Here's how the part is built. I have some questions about the finished solid (model axes, mm). A direction names the side the tool comes from. Give positions to 0.01 mm unless a question says otherwise; leave off trailing zeros. Order: outer loops, then holes, each group sorted by start corner. A loop starts at its lowest first (then second) coordinate and runs counter-clockwise, first axis right, second up. Notation, with made-up numbers: (-40, 61) -> (5, 61) arc R20 cw to (5, 69) -> close; hole circle Ø11 at (0.25, -12). An arc over 180 degrees is marked (long way). Write each question's results on one line, items separated by ' | '. Start each with the question number.
Q1. Thinking about a two-plate mould opening in X: for faces 4 (the face through (-13.715, -4, -7)), 5 (the face through (5, -33.779, -7)), 6 (the face through (5, 27.921, -7)), 7 (the face through (16, -23, 0)), which applies, pulls with the +X half, pulls with the -X half, needs draft (parallel to the pull), parting line crosses it, or undercut?
Q2. I need wall thicknesses on line 1 along Y through (x, z) = (16, -3.25); line 2 along X through (y, z) = (-27, -8.25); line 3 along Y through (x, z) = (7, -3.25). Which ranges of each line are inside material? Lowest first, please. Write a range as [from, to].
Q3. For faces 1 (the face through (14.75, -26.114, 1.507)), 2 (the face through (5, -35.779, -7)), 3 (the face through (20.585, -4, -7)), which set-ups out of +Z, -Z, +X, -X, +Y, -Y let a thin tool reach every point of the face, with its end or its side?
Q4. I'm going to push flat-ended pins straight in: pin 1 (1.4 mm diameter, centred on x = -6, y = 22.5, fed in from -Z); pin 2 (1.4 mm diameter, centred on x = -7, y = -24, fed in from +Z); pin 3 (3 mm diameter, centred on x = 14, y = 13, fed in from -Z). Where does each tip first touch, or does it pass through?
Q5. Imagine slicing it at B-B, the plane z = -5.75. Please give me the cut outline in (x, y).
Q6. Imagine slicing it at D-D, the plane y = -1. Please give me the cut outline in (x, z), then the cut area to 3 significant figures.
```python
from build123d import *

# Parameters (mm, degrees)
CROQUIS1_W              = 36.3
CROQUIS1_H              = 63.7
SALIENTE_EXTRUIR1_DEPTH = 2
CROQUIS2_R              = 1.45
CORTAR_EXTRUIR1_DEPTH   = 43.35833467
CROQUIS3_W              = 36.3
CROQUIS3_H              = 63.7
CROQUIS3_W_2            = 32.3
CROQUIS3_H_2            = 59.7
SALIENTE_EXTRUIR2_DEPTH = 15
CROQUIS4_W              = 8.458215844
CROQUIS4_H              = 3.322323253
CORTAR_EXTRUIR2_DEPTH   = 15
CROQUIS5_W              = 10.947551138
CROQUIS5_H              = 4.889557179
CORTAR_EXTRUIR3_DEPTH   = 1
CROQUIS6_R              = 2.4
SALIENTE_EXTRUIR3_DEPTH = 10
REDONDEO1_R             = 1
CORTAR_EXTRUIR4_DEPTH   = 1


with BuildPart() as part:
    # Croquis1 → Saliente-Extruir1 (new body)
    with BuildSketch(Plane.XY):
        with Locations((4.435020115, -3.929119363)):
            Rectangle(CROQUIS1_W, CROQUIS1_H)
    extrude(amount=SALIENTE_EXTRUIR1_DEPTH)

    # Croquis2 → Cortar-Extruir1 (cut, through all)
    with BuildSketch(Plane(origin=(0, 0, 0), x_dir=(-1, 0, 0), z_dir=(0, 0, -1))):
        with Locations((-16.185020115, 23.120880637)):
            Circle(CROQUIS2_R)
        with Locations((7.314979885, 23.120880637)):
            Circle(CROQUIS2_R)
        with Locations((7.314979885, -23.479119363)):
            Circle(CROQUIS2_R)
        with Locations((-16.185020115, -23.479119363)):
            Circle(CROQUIS2_R)
    extrude(amount=-CORTAR_EXTRUIR1_DEPTH, mode=Mode.SUBTRACT)

    # Croquis3 → Saliente-Extruir2 (add)
    with BuildSketch(Plane(origin=(0, 0, 0), x_dir=(-1, 0, 0), z_dir=(0, 0, -1))):
        with Locations((-4.435020115, -3.929119363)):
            Rectangle(CROQUIS3_W, CROQUIS3_H)
        with Locations((-4.435020115, -3.929119363)):
            Rectangle(CROQUIS3_W_2, CROQUIS3_H_2, mode=Mode.SUBTRACT)
    extrude(amount=SALIENTE_EXTRUIR2_DEPTH)

    # Croquis4 → Cortar-Extruir2 (cut)
    with BuildSketch(Plane(origin=(0, 27.920880637, 0), x_dir=(1, 0, 0), z_dir=(0, 1, 0))):
        with Locations((4.530912193, 12.938838374)):
            Rectangle(CROQUIS4_W, CROQUIS4_H)
    extrude(amount=-CORTAR_EXTRUIR2_DEPTH, mode=Mode.SUBTRACT)

    # Croquis5 → Cortar-Extruir3 (cut)
    with BuildSketch(Plane(origin=(0, 27.920880637, 0), x_dir=(1, 0, 0), z_dir=(0, 1, 0))):
        with Locations((4.498418707, 12.555221411)):
            Rectangle(CROQUIS5_W, CROQUIS5_H)
    extrude(amount=-CORTAR_EXTRUIR3_DEPTH, mode=Mode.SUBTRACT)

    # Croquis6 → Saliente-Extruir3 (add)
    with BuildSketch(Plane(origin=(0, 0, 0), x_dir=(-1, 0, 0), z_dir=(0, 0, -1))):
        with Locations(Location((-16.185020115, 23.120880637, 0), (0, 0, 180))):
            Circle(CROQUIS6_R)
        with Locations(Location((7.314979885, 23.120880637, 0), (0, 0, 180))):
            Circle(CROQUIS6_R)
        with Locations(Location((7.314979885, -23.479119363, 0), (0, 0, 180))):
            Circle(CROQUIS6_R)
        with Locations(Location((-16.185020115, -23.479119363, 0), (0, 0, 180))):
            Circle(CROQUIS6_R)
    extrude(amount=SALIENTE_EXTRUIR3_DEPTH)

    # Redondeo1
    redondeo1_edges = [part.edges().sort_by_distance(p)[0] for p in [
        (-0.975356862, 27.920880637, -12.55522141),
        (4.498418707, 27.920880637, -10.110442821),
        (9.972194276, 27.920880637, -12.55522141),
        (22.585020115, -3.929119363, 2),
        (22.585020115, -35.779119363, -6.5),
        (4.435020115, -35.779119363, 2),
        (-13.714979885, -35.779119363, -6.5),
        (-13.714979885, -3.929119363, 2),
        (4.435020115, 27.920880637, 2),
        (-13.714979885, 27.920880637, -6.5),
        (22.585020115, 27.920880637, -6.5),
    ]]
    fillet(redondeo1_edges, radius=REDONDEO1_R - 0.0001)  # a hair under: the kernel refuses the full size

    # Croquis7 → Cortar-Extruir4 (cut)
    with BuildSketch(Plane.XY.offset(2)):
        Polygon((-5.626866213, 20.095938946), (-3.8512467, 23.070359116), (-5.539360372, 26.095300806), (-9.003093557, 26.145822327), (-10.77871307, 23.171402157), (-9.090599398, 20.146460467), align=None)
        Polygon((17.887203126, 20.103833571), (19.648951024, 23.086490833), (17.946768013, 26.103537899), (14.482837104, 26.137927702), (12.721089206, 23.15527044), (14.423272217, 20.138223374), align=None)
        Polygon((-4.386581268, -25.329654838), (-4.248169845, -21.868319506), (-7.176568462, -20.017784032), (-10.243378502, -21.628583889), (-10.381789925, -25.089919221), (-7.453391308, -26.940454695), align=None)
        Polygon((19.240442153, -25.111417183), (19.126342512, -21.649195169), (16.070920474, -20.01689735), (13.129598077, -21.846821544), (13.243697718, -25.309043558), (16.299119756, -26.941341377), align=None)
    extrude(amount=-CORTAR_EXTRUIR4_DEPTH, mode=Mode.SUBTRACT)


solid = part.part
```
Geometry check:
1) face 4: pulls with the -X half | face 5: undercut | face 6: needs draft | face 7: undercut
2) line 1: [-35.78, -33.78], [-25.87, -21.09], [20.73, 25.51], [25.92, 27.92] | line 2: [-13.71, -11.71], [20.59, 22.59] | line 3: [-35.78, -33.78], [25.92, 27.92]
3) face 1: +Z | face 2: +Z, -Z, +X, -X, -Y | face 3: -Z
4) pin 1: z = -10 | pin 2: z = 0 | pin 3: z = 0
5) outline: (-13.71, -34.78) arc R1 ccw to (-12.72, -35.78) -> (21.59, -35.78) arc R1 ccw to (22.59, -34.78) -> (22.59, 26.92) arc R1 ccw to (21.59, 27.92) -> (-12.72, 27.92) arc R1 ccw to (-13.71, 26.92) -> close; circle Ø4.8 at (-7.31, -23.48); circle Ø4.8 at (-7.31, 23.12); circle Ø4.8 at (16.19, -23.48); circle Ø4.8 at (16.19, 23.12); hole (-11.71, -33.78) -> (20.59, -33.78) -> (20.59, 25.92) -> (-11.71, 25.92) -> close
6) outline: (-13.71, -15) -> (-11.71, -15) -> (-11.71, 0) -> (20.59, 0) -> (20.59, -15) -> (22.59, -15) -> (22.59, 1) arc R1 ccw to (21.59, 2) -> (-12.72, 2) arc R1 ccw to (-13.71, 1) -> close | area: 132 mm²
